Check sheet for the drawn part. Datum: minimum x, y, z corner. Units: mm. Give positions to 0.01 mm unless a question says otherwise; leave off trailing zeros. Loops run counter-clockwise (first coordinate to the right, second up) from the corner with the lowest first, then second, coordinate; pieces in that order, holes last. Notation, with made-up numbers: (43.5, 80) - (94.5, 80) arc R24 ccw to (94.5, 104) - close; hole circle Ø8 at (-28.5, 29.5). An arc over 180 degrees is marked (long way). Answer in a Markdown table with one row per item.
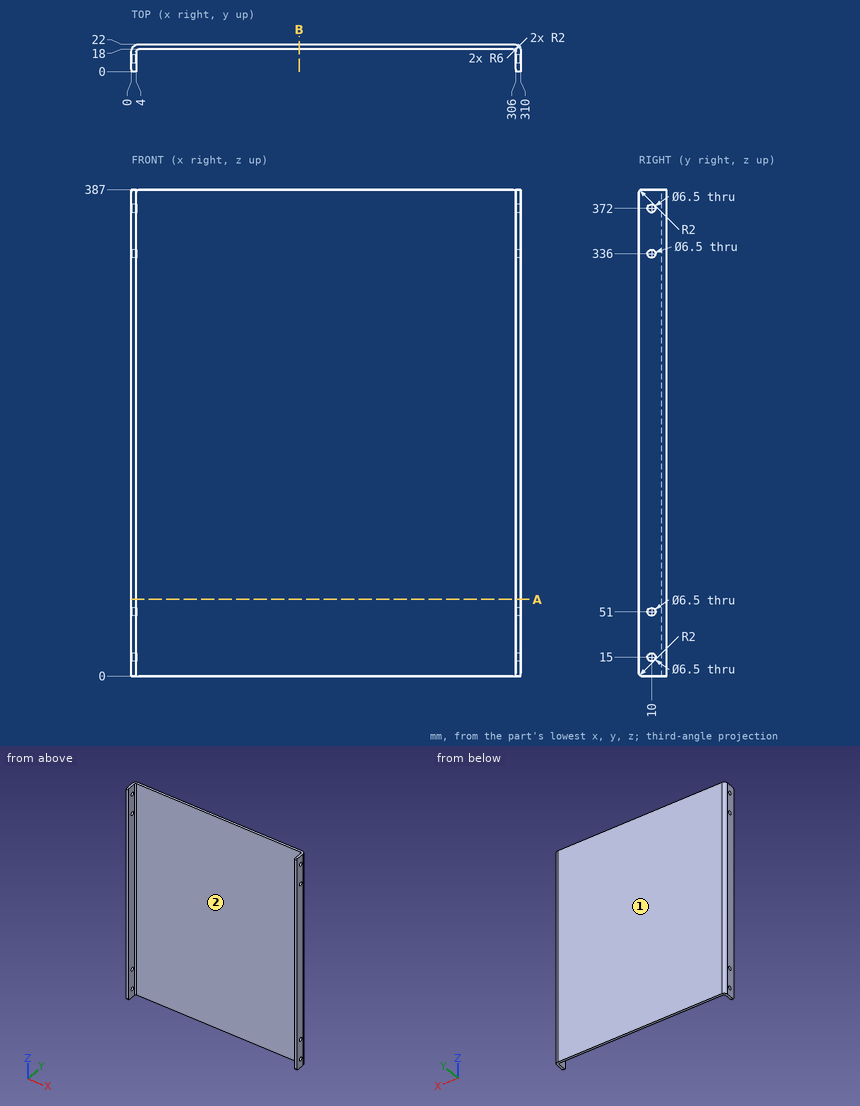
Q1. Go/stop test with flat-tipped pins: P1, Ø1, axis at y = 17, z = 80.5, coming from the -X side; P2, Ø1.5, axis at x = 227.5, z = 340, coming from the -Y side. Record where each tip stops, or that it passes through.
Completed:
| item | result |
|---|---|
| P1 | x = 0.02 |
| P2 | y = 18 |
Q2. Thickness scan on line 1 (X direction, y = 1.5, z = 263); line 2 (Y direction, x = 133.5, z = 191); line 3 (Y direction, x = 307, z = 15). Record the ranges inside material, lowest first.
Completed:
| item | result |
|---|---|
| line 1 | 0 to 4, 306 to 310 |
| line 2 | 18 to 22 |
| line 3 | 0 to 6.75, 13.25 to 21.2 |
Q3. Sectioned sample at B-B (x = 133.5). Record the cut outline in (y, z), and give its area (3 significant figures).
Completed:
| item | result |
|---|---|
| outline | (18, 0) - (22, 0) - (22, 387) - (18, 387) - close |
| area | 1,550 mm^2 |
Q4. Draft check along X on the marked faces 1 and 2. Enter one of: +X half, -X half, draft (parallel to the pull), parting line (faces both ways), or undercut.
Completed:
| item | result |
|---|---|
| face 1 | draft |
| face 2 | undercut |
Q5. Sectioned sample at A-A (z = 61). Record the cut outline in (x, y).
Completed:
| item | result |
|---|---|
| outline | (0, 0) - (4, 0) - (4, 16) arc R2 cw to (6, 18) - (304, 18) arc R2 cw to (306, 16) - (306, 0) - (310, 0) - (310, 16) arc R6 ccw to (304, 22) - (6, 22) arc R6 ccw to (0, 16) - close |
